CAD build for the part. Positions are in the model's coordinates, mm. A direction names the side the tool comes from. Round coordinates to 2 decimals unless told otherwise and drop trailing zeros. Loops run counter-clockwise (first coordinate to the right, second up) from the corner with the lowest first, then second, coordinate; pieces in that order, holes last. Notation, with made-up numbers: M 38.25,19 L 46.25,19 A26 ccw 46.25,37 Z; hole C -34.5,-36.5 d8. An arc over 180 degrees is marked long. Put each result on its own line as item: value. Start each with the question number.
from build123d import *

# Parameters (mm, degrees)
RESSALTO_EXTRUS_O1_DEPTH = 25
ESBO_O2_R                = 1.05
CORTE_EXTRUS_O1_DEPTH    = 20
ESBO_O3_R                = 2.5
CORTE_EXTRUS_O3_DEPTH    = 2.5


with BuildPart() as part:
    # Esboço1 → Ressalto-extrusão1 (new body)
    with BuildSketch(Plane(origin=(0, 0, 0), x_dir=(0, 1, 0), z_dir=(0, 0, 1))):
        Polygon((-6, 0), (6, 0), (4, 5), (-4, 5), align=None)
    extrude(amount=RESSALTO_EXTRUS_O1_DEPTH)

    # Esboço2 → Corte-extrusão1 (cut)
    with BuildSketch(Plane.YZ):
        with Locations(Location((0, 20, 0), (0, 0, 270))):
            Circle(ESBO_O2_R)
        with Locations(Location((0, 5, 0), (0, 0, 270))):
            Circle(ESBO_O2_R)
    extrude(amount=-CORTE_EXTRUS_O1_DEPTH, mode=Mode.SUBTRACT)

    # Esboço3 → Corte-extrusão3 (cut)
    with BuildSketch(Plane.YZ):
        with Locations(Location((0, 20, 0), (0, 0, 270))):
            Circle(ESBO_O3_R)
        with Locations(Location((0, 5, 0), (0, 0, 270))):
            Circle(ESBO_O3_R)
    extrude(amount=-CORTE_EXTRUS_O3_DEPTH, mode=Mode.SUBTRACT)


solid = part.part
(1) Cut at D-D on y = -1.5. List the corners of the cut face in (x, z), and give its area (3 significant figures).
(2) Cut at A-A on y = 0. List the corners of the cut face in (x, z), and give its area (3 significant figures).
(3) Mould opens along Z. For faces 1 (the flat face through (-2.5, -1, 4)), 2 (the flat face through (0, 0, 12)), 3 (the flat face through (-3, 0, 25)) say: +Z half, -Z half, draft (parallel to the pull), parting line (faces both ways), or undercut.
(4) Tool access for faces 4 (the cylindrical face through (-1.2, 0.1, 22.5)), 5 (the cylindrical face through (-3.73, 0.05, 21.05)): list every direction of +Z, -Z, +X, -X, +Y, -Y with a clear straight run to the whole face (end or side of a thin tool).
(5) Drill centre lines: line 1 along Z through (x, y) = (-2.3, 0.25); line 2 along Z through (x, y) = (-2, 0.75); line 3 along Y through (x, z) = (-1.3, 5). Where is each one in solid material? Low to high.
(6) Flat gauge pins, fed straight in: pin 1 Ø3 at (y, z) = (-4.5, 14.5) entering from -X; pin 2 Ø4.5 at (y, z) = (0, 20) entering from +X; pin 3 Ø2 at (x, z) = (-2, 3.5) entering from -Y. Where does each tip first touch, or does it go through?
(7) Cut at B-B on z = 20. List the corners of the cut face in (x, y).
(8) Cut at C-C on x = -4.65. List the corners of the cut face in (y, z), and give its area (3 significant figures).
Taken from the geometry:
1. outline: M -5,0 L 0,0 L 0,3 L -2.5,3 L -2.5,7 L 0,7 L 0,18 L -2.5,18 L -2.5,22 L 0,22 L 0,25 L -5,25 Z
1. area: 105 mm2
2. outline: M -5,0 L 0,0 L 0,2.5 L -2.5,2.5 L -2.5,3.95 L -5,3.95 Z; M -5,6.05 L -2.5,6.05 L -2.5,7.5 L 0,7.5 L 0,17.5 L -2.5,17.5 L -2.5,18.95 L -5,18.95 Z; M -5,21.05 L -2.5,21.05 L -2.5,22.5 L 0,22.5 L 0,25 L -5,25 Z
2. area: 89.5 mm2
3. face 1: undercut
3. face 2: draft
3. face 3: +Z half
4. face 4: +X
4. face 5: +X, -X
5. line 1: 0 to 2.51, 7.49 to 17.51, 22.49 to 25
5. line 2: 0 to 2.62, 7.38 to 17.62, 22.38 to 25
5. line 3: -5.48 to -2.5, 2.5 to 5.48
6. pin 1: x = -5
6. pin 2: x = -2.5
6. pin 3: y = -5.6
7. outline: M -5,-4 L 0,-6 L 0,-2.5 L -2.5,-2.5 L -2.5,-1.05 L -5,-1.05 Z; M -5,1.05 L -2.5,1.05 L -2.5,2.5 L 0,2.5 L 0,6 L -5,4 Z
8. outline: M -4.14,0 L 4.14,0 L 4.14,25 L -4.14,25 Z; hole C 0,5 d2.1; hole C 0,20 d2.1
8. area: 200 mm2
